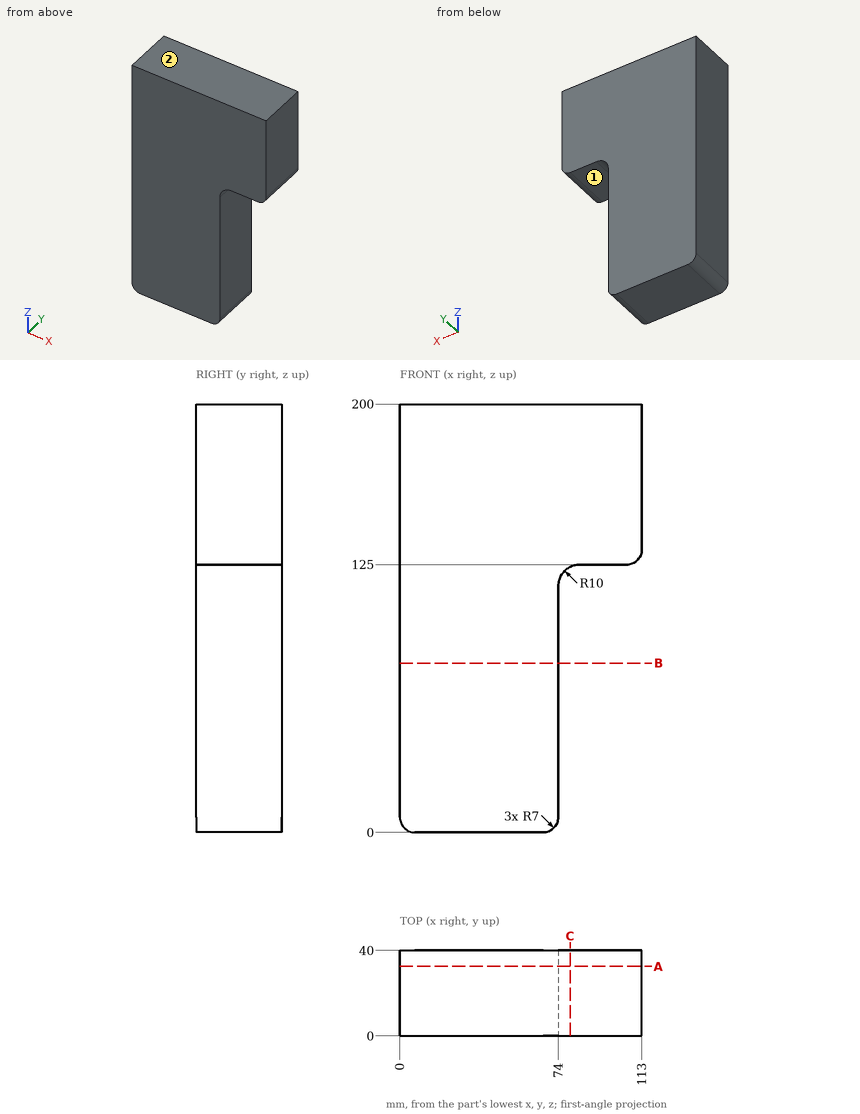
Here's the drawing with two shaded views (mm, measured from the low corner). I have some questions. A direction names the side the tool comes from. Round coordinates to 2 decimals unless told otherwise and drop trailing zeros. Loops run counter-clockwise (first coordinate to the right, second up) from the corner with the lowest first, then second, coordinate; pieces in that order, holes last. Notation, with made-up numbers: (76, 78.25) - (128, 78.25) arc R25 ccw to (128, 98.25) - close; hole circle Ø1 at (42, 11.25). An arc over 180 degrees is marked (long way). Write item = value, one per line.
1) Imagine slicing it at B-B (z = 79). Please give me the cut outline in (x, y), and give its area (3 significant figures).
Computed:
outline = (0, 0) - (74, 0) - (74, 40) - (0, 40) - close
area = 2,960 mm2
2) I'm going to push flat-ended pins straight in: P1, Ø11, axis at x = 99.5, y = 10.5, coming from the -Z side; P2, Ø20, axis at y = 17, z = 85.5, coming from the +X side. Where does each tip first touch, or does it pass through?
Computed:
P1 = 125
P2 = 74
3) Imagine slicing it at C-C (x = 79.5). Please give me the cut outline in (y, z).
Computed:
outline = (0, 123.93) - (40, 123.93) - (40, 200) - (0, 200) - close
4) On a 3-axis mill with a long thin cutter (end or side, diameter ignored), from which of +Z, -Z, +X, -X, +Y, -Y can I reach the whole of each face in a straight line? I mean the marked faces 1 and 2. Say none if no direction works.
Computed:
face_1 = -Z, +X, +Y, -Y
face_2 = +Z, +X, -X, +Y, -Y
5) I need wall thicknesses on line 1 along X through (y, z) = (36, 108); line 2 along X through (y, z) = (20, 124); line 3 along Z through (x, y) = (71, 12). Which ranges of each line are inside material? Lowest first, please. Write a range as from..to.
Computed:
line_1 = 0..74
line_2 = 0..79.64
line_3 = 1.26..200
6) Imagine slicing it at A-A (y = 32.5). Please give me the cut outline in (x, z), and give its area (3 significant figures).
Computed:
outline = (0, 7) arc R7 ccw to (7, 0) - (67, 0) arc R7 ccw to (74, 7) - (74, 115) arc R10 cw to (84, 125) - (106, 125) arc R7 ccw to (113, 132) - (113, 200) - (0, 200) - close
area = 17,700 mm2
